The listing builds one solid part. Answer for the finished solid, in the listing's coordinates (mm). Face numbers are marked on the shaded views. Give positions to 0.01 mm unless a question says otherwise; leave off trailing zeros. Loops run counter-clockwise (first coordinate to the right, second up) from the corner with the lowest first, then second, coordinate; pieces in that order, holes last. Notation, with made-up numbers: (27.25, 49) - (65.25, 49) arc R27 cw to (65.25, 70) - close; hole circle Ø11 at (3.25, -8). An arc over 180 degrees is marked (long way). One line per item, written item: value. Start each with the question number.
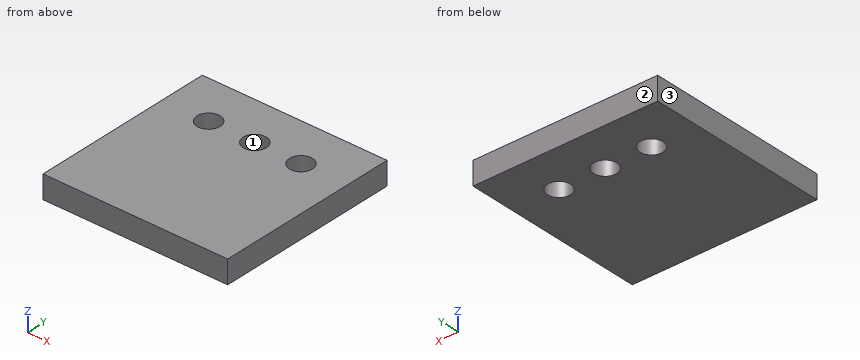
Autodesk Inventor part; units mm, degrees
ref_plane "YZ Plane" through (0, 0, 0) normal (1, 0, 0) x (0, 1, 0)
ref_plane "XZ Plane" through (0, 0, 0) normal (0, 1, 0) x (-1, 0, 0)
ref_plane "XY Plane" through (0, 0, 0) normal (0, 0, 1) x (1, 0, 0)
sketch "Sketch1" plane through (0, 0, 0) normal (0, 0, 1) x (1, 0, 0)
  line L0 (0, 0) -> (-50.8, 0)
  line L1 (-50.8, 0) -> (-50.8, 50.8)
  line L2 (-50.8, 50.8) -> (0, 50.8)
  line L3 (0, 50.8) -> (0, 0)
  dimension "d0" = 50.8
  dimension "d1" = 50.8
extrude "Extrusion1" add sketch "Sketch1" along normal blind 6.35
sketch "Sketch2" plane through (0, 0, 6.35) normal (0, 0, 1) x (1, 0, 0)
  line L0 (0, 50.8) -> (0, 0)
  line L1 (-50.8, 50.8) -> (0, 50.8)
  circle A0 centre (-12.7, 38.1) radius 3.175
  dimension "d4" = 12.7
  dimension "d5" = 12.7
  dimension "d6" = 6.35
extrude "Extrusion2" cut sketch "Sketch2" against normal through all
pattern_linear "Rectangular Pattern1" count 3 spacing 12.7 along (-1, 0, 0) of "Extrusion2"
properties part number "Shovel_PivotMount" material "Aluminum-6061"
1. Determine the mould class of the marked faces 1, 2 and 3 for opening direction Y: released by +Y, released by -Y, zero draft, split by the parting line, or undercut.
2. A cutting plane is placed at A-A (x = -12.7). Determine the outline of the cut face in (y, z) (3 decimals), plus the area to 3 significant figures.
3. A cutting plane is placed at C-C (y = 38.1). Determine the outline of the cut face in (x, z) (3 decimals), plus the area to 3 significant figures.
4. A cutting plane is placed at B-B (z = 4.25). Determine the outline of the cut face in (x, y) (3 decimals).
5. A cutting plane is placed at D-D (x = -25). Determine the outline of the cut face in (y, z).
6. Find the intervals of material crossed by L1, parallel to Y at x = -12.7, z = 3 (3 decimals); L2, parallel to X at y = 38.5, z = 2.25; L3, parallel to X at y = 36.5, z = 4.75, in increasing order. Write a range as [from, to].
Results below:
1. face 1: undercut
1. face 2: released by +Y
1. face 3: zero draft
2. outline: (0, 0) - (34.925, 0) - (34.925, 6.35) - (0, 6.35) - close; (41.275, 0) - (50.8, 0) - (50.8, 6.35) - (41.275, 6.35) - close
2. area: 282 mm^2
3. outline: (-50.8, 0) - (-41.275, 0) - (-41.275, 6.35) - (-50.8, 6.35) - close; (-34.925, 0) - (-28.575, 0) - (-28.575, 6.35) - (-34.925, 6.35) - close; (-22.225, 0) - (-15.875, 0) - (-15.875, 6.35) - (-22.225, 6.35) - close; (-9.525, 0) - (0, 0) - (0, 6.35) - (-9.525, 6.35) - close
3. area: 202 mm^2
4. outline: (-50.8, 0) - (0, 0) - (0, 50.8) - (-50.8, 50.8) - close; hole circle Ø6.35 at (-38.1, 38.1); hole circle Ø6.35 at (-25.4, 38.1); hole circle Ø6.35 at (-12.7, 38.1)
5. outline: (0, 0) - (34.95, 0) - (34.95, 6.35) - (0, 6.35) - close; (41.25, 0) - (50.8, 0) - (50.8, 6.35) - (41.25, 6.35) - close
6. L1: y = [0, 34.925], [41.275, 50.8]
6. L2: x = [-50.8, -41.25], [-34.95, -28.55], [-22.25, -15.85], [-9.55, 0]
6. L3: x = [-50.8, -40.84], [-35.36, -28.14], [-22.66, -15.44], [-9.96, 0]
